from build123d import *

# Parameters (mm, degrees)
BOSS_EXTRUDE1_DEPTH     = 10
CUT_EXTRUDE1_DEPTH      = 29.705400189
CUT_EXTRUDE1_DEPTH_BACK = 29.705400189
SKETCH2_R               = 1.55


with BuildPart() as part:
    # Sketch1 → Boss-Extrude1 (new, symmetric)
    with BuildSketch(Plane.XY):
        Polygon((-3, 20), (-3, 0), (3, 0), (3, 20), (8, 20), (8, 0), (18, 0), (18, -5), (-18, -5), (-18, 0), (-8, 0), (-8, 20), align=None)
    extrude(amount=BOSS_EXTRUDE1_DEPTH, both=True)

    # Sketch2 → Cut-Extrude1 (cut, two sides: drawn at the far end of the back side and taken through both)
    with BuildSketch(Plane(origin=(0, 0, 0), x_dir=(0, 0, -1), z_dir=(1, 0, 0)).offset(-CUT_EXTRUDE1_DEPTH_BACK)):
        with Locations(Location((0, 10, 0), (0, 0, 270))):
            Circle(SKETCH2_R)
    extrude(amount=CUT_EXTRUDE1_DEPTH + CUT_EXTRUDE1_DEPTH_BACK, mode=Mode.SUBTRACT)


solid = part.part
Could you check a few things on this model? Use its own coordinates, in mm. A direction names the side the tool comes from. Coordinates: 2 decimals unless noted, no trailing zeros. Loops run counter-clockwise (first coordinate to the right, second up) from the corner with the lowest first, then second, coordinate; pieces in that order, holes last.
1. Imagine slicing it at C-C (z = 3.25). Please give me the cut outline in (x, y).
2. We'd pull the mould along X, two halves only. Please class faces 4 (the face through (18, -2, 0)), 5 (the face through (0, 0, 0)), 6 (the face through (0, -5, 0)): released by +X, released by -X, zero draft, split by the parting line, or undercut.
3. Imagine slicing it at A-A (z = 0). Please give me the cut outline in (x, y), and give its area (3 significant figures).
4. For faces 1 (the face through (-13, 0, 0)), 2 (the face through (8, 12, 0)), 3 (the face through (3, 12, 0)), which set-ups out of +Z, -Z, +X, -X, +Y, -Y let a thin tool reach every point of the face, with its end or its side?
5. I need wall thicknesses on L1, parallel to Z at x = -4.45, y = 10; L2, parallel to X at y = 17.5, z = -7.5; L3, parallel to Y at x = -8.5, z = -3. Which ranges of each line are inside material? Lowest first, please.
6. For P1, Ø3, axis at y = 10, z = 0, coming from the -X side; P2, Ø5, axis at y = 16, z = 1.5, coming from the -X side; P3, Ø3, axis at x = -11.5, z = 4, coming from the +Y side, each with a flat end and sliding along its axis, tell me the tip position at first contact or that it passes through.
7. Imagine slicing it at B-B (y = 8). Please give me the cut outline in (x, z), and give its area (3 significant figures).
8. Imagine slicing it at D-D (x = 3.5). Please give me the cut outline in (y, z).
Computed values:
1. outline: (-18, -5) - (18, -5) - (18, 0) - (8, 0) - (8, 20) - (3, 20) - (3, 0) - (-3, 0) - (-3, 20) - (-8, 20) - (-8, 0) - (-18, 0) - close
2. face 4: released by +X
2. face 5: undercut
2. face 6: zero draft
3. outline: (-18, -5) - (18, -5) - (18, 0) - (8, 0) - (8, 8.45) - (3, 8.45) - (3, 0) - (-3, 0) - (-3, 8.45) - (-8, 8.45) - (-8, 0) - (-18, 0) - close; (-8, 11.55) - (-3, 11.55) - (-3, 20) - (-8, 20) - close; (3, 11.55) - (8, 11.55) - (8, 20) - (3, 20) - close
3. area: 349 mm2
4. face 1: +Z, -Z, -X, +Y
4. face 2: +Z, -Z, +X, +Y
4. face 3: +Z, -Z, +Y
5. L1: z = -10 to -1.55, 1.55 to 10
5. L2: x = -8 to -3, 3 to 8
5. L3: y = -5 to 0
6. P1: passes through
6. P2: stops at x = -8
6. P3: stops at y = 0
7. outline: (-8, -10) - (-3, -10) - (-3, 10) - (-8, 10) - close; (3, -10) - (8, -10) - (8, 10) - (3, 10) - close
7. area: 200 mm2
8. outline: (-5, -10) - (20, -10) - (20, 10) - (-5, 10) - close; hole circle Ø3.1 at (10, 0)
